```python
from build123d import *

# Parameters (mm, degrees)
ESQUISSE1_R             = 8
BOSS_EXTRU_1_DEPTH      = 18
ESQUISSE2_R             = 8.85
BOSS_EXTRU_2_DEPTH      = 1.5
ESQUISSE3_R             = 7
ENL_V_MAT_EXTRU_1_DEPTH = 1
ESQUISSE4_R             = 7.5
BOSS_EXTRU_3_DEPTH      = 8.5
ESQUISSE5_W             = 0.6
ESQUISSE5_H             = 3
ESQUISSE5_W_2           = 3
ESQUISSE5_H_2           = 0.6
BOSS_EXTRU_4_DEPTH      = 6
BOSS_EXTRU_5_START      = 9
BOSS_EXTRU_5_DEPTH      = 2.9


with BuildPart() as part:
    # Esquisse1 → Boss.-Extru.1 (new body)
    with BuildSketch(Plane(origin=(0, 0, 0), x_dir=(1, 0, 0), z_dir=(0, 1, 0))):
        with Locations(Location((0, 0, 0), (0, 0, 270))):
            Circle(ESQUISSE1_R)
    extrude(amount=-BOSS_EXTRU_1_DEPTH)

    # Esquisse2 → Boss.-Extru.2 (add)
    with BuildSketch(Plane(origin=(0, 0, 0), x_dir=(1, 0, 0), z_dir=(0, 1, 0))):
        with Locations(Location((0, 0, 0), (0, 0, 270))):
            Circle(ESQUISSE2_R)
    extrude(amount=BOSS_EXTRU_2_DEPTH)

    # Esquisse3 → Enlèv. mat.-Extru.1 (cut)
    with BuildSketch(Plane(origin=(0, 1.5, 0), x_dir=(1, 0, 0), z_dir=(0, 1, 0))):
        with Locations(Location((0, 0, 0), (0, 0, 270))):
            Circle(ESQUISSE3_R)
        with BuildLine():
            Line((-0.8, 0), (-0.8, 4.75466628))
            ThreePointArc((-0.8, 4.75466628), (0, 5.55466628), (0.8, 4.75466628))
            Line((0.8, 4.75466628), (0.8, 0))
            ThreePointArc((0.8, 0), (0, -0.8), (-0.8, 0))
        make_face(mode=Mode.SUBTRACT)
        with BuildLine():
            ThreePointArc((-2.913082643, 3.814963894), (0, -4.8), (2.913082643, 3.814963894))
            ThreePointArc((2.913082643, 3.814963894), (1.791741554, 3.664650352), (1.942055095, 2.543309263))
            ThreePointArc((1.942055095, 2.543309263), (0, -3.2), (-1.942055095, 2.543309263))
            ThreePointArc((-1.942055095, 2.543309263), (-1.791741554, 3.664650352), (-2.913082643, 3.814963894))
        make_face(mode=Mode.SUBTRACT)
    extrude(amount=-ENL_V_MAT_EXTRU_1_DEPTH, mode=Mode.SUBTRACT)

    # Esquisse4 → Boss.-Extru.3 (add)
    with BuildSketch(Plane.XZ.offset(18)):
        with Locations(Location((0, 0, 0), (0, 0, 270))):
            Circle(ESQUISSE4_R)
    extrude(amount=BOSS_EXTRU_3_DEPTH)

    # Esquisse5 → Boss.-Extru.4 (add)
    with BuildSketch(Plane.XZ.offset(26.5)):
        with Locations((-4.616296437, -1.823639602)):
            Rectangle(ESQUISSE5_W, ESQUISSE5_H)
        with Locations((0, 5.19973439)):
            Rectangle(ESQUISSE5_W_2, ESQUISSE5_H_2)
        with Locations((4.616296437, -1.823639602)):
            Rectangle(ESQUISSE5_W, ESQUISSE5_H)
        with Locations((0, 0.93263523)):
            Rectangle(ESQUISSE5_W_2, ESQUISSE5_H_2)
        with Locations((-0.5, -5.623689166)):
            Rectangle(ESQUISSE5_W_2, ESQUISSE5_H_2)
    extrude(amount=BOSS_EXTRU_4_DEPTH)

    # Esquisse6 → Boss.-Extru.5 (add)
    with BuildSketch(Plane.XZ.offset(BOSS_EXTRU_5_START)):
        Polygon((10.911920088, 0), (5.455960044, 9.45), (-5.455960044, 9.45), (-10.911920088, 0), (-5.455960044, -9.45), (5.455960044, -9.45), align=None)
    extrude(amount=BOSS_EXTRU_5_DEPTH)


solid = part.part
```
Can you work these out from the model? Positions are in its coordinate system, mm. A direction names the side the tool comes from. Coordinates: 2 decimals unless noted, no trailing zeros. Loops run counter-clockwise (first coordinate to the right, second up) from the corner with the lowest first, then second, coordinate; pieces in that order, holes last.
1) Imagine slicing it at A-A on y = -10.5. List the corners of the cut face in (x, z) for me.
2) Imagine slicing it at B-B on x = 6.5. List the corners of the cut face in (y, z) for me.
3) I need wall thicknesses on probe 1 along X at (y, z) = (-29, -0.75); probe 2 along Y at (x, z) = (-0.5, -8.5); probe 3 along Z at (x, y) = (-0.25, -3). Which ranges of each line are inside material? Lowest first, please.
4) Which directions (+Z, -Z, +X, -X, +Y, -Y) give clear straight access to the entire face, cutting with the end or side of a thin tool? Please do faces 1 (the flat face through (-5, 0, -7)), 2 (the flat face through (4.316, -29, -2)), 3 (the flat face through (0, -29, 5.5)), 4 (the flat face through (-0.8, 1, -2)), 5 (the flat face through (4.916, -29, -2)).
5) Thinking about a two-plate mould opening in Y: for faces 6 (the flat face through (-1, 1.5, 3.3)), 7 (the flat face through (-8.146, -10.43, 4.791)), 8 (the cylindrical face through (-7.81, -4.44, -1.73)), which applies, pulls with the +Y half, pulls with the -Y half, needs draft (parallel to the pull), parting line crosses it, or undercut?
6) Imagine slicing it at C-C on y = -19. List the corners of the cut face in (x, z) for me, plus the area to 3 significant figures.
7) For pin 1 (0.7 mm diameter, centred on y = -30.5, z = 5, fed in from -X); pin 2 (1.5 mm diameter, centred on x = -0.5, y = -28.5, fed in from +Z); pin 3 (0.5 mm diameter, centred on x = -4.5, y = -30, fed in from -Z), each with a flat end and sliding along its axis, tell me the tip position at first contact or that it passes through.
Completed:
1. outline: (-10.91, 0) - (-5.46, -9.45) - (5.46, -9.45) - (10.91, 0) - (5.46, 9.45) - (-5.46, 9.45) - close
2. outline: (-26.5, -3.74) - (-18, -3.74) - (-18, -4.66) - (-11.9, -4.66) - (-11.9, -7.64) - (-9, -7.64) - (-9, -4.66) - (0, -4.66) - (0, -6.01) - (1.5, -6.01) - (1.5, -2.6) - (0.5, -2.6) - (0.5, 2.6) - (1.5, 2.6) - (1.5, 6.01) - (0, 6.01) - (0, 4.66) - (-9, 4.66) - (-9, 7.64) - (-11.9, 7.64) - (-11.9, 4.66) - (-18, 4.66) - (-18, 3.74) - (-26.5, 3.74) - close
3. probe 1: x = -4.92 to -4.32, 4.32 to 4.92
3. probe 2: y = -11.9 to -9, 0 to 1.5
3. probe 3: z = -8 to 8
4. face 1: none
4. face 2: +Z, -Z, -Y
4. face 3: +Z, +X, -X, -Y
4. face 4: +Y
4. face 5: +Z, -Z, +X, -Y
5. face 6: pulls with the +Y half
5. face 7: needs draft
5. face 8: undercut
6. outline: circle Ø15 at (0, 0)
6. area: 177 mm2
7. pin 1: stops at x = -1.5
7. pin 2: stops at z = 5.5
7. pin 3: stops at z = -3.32
